Part model, mm, in its own coordinate system. Face numbers are marked on the shaded views. A direction names the side the tool comes from. Give positions to 0.01 mm unless a question says otherwise; leave off trailing zeros. Order: outer loops, then holes, each group sorted by start corner. A loop starts at its lowest first (then second) coordinate and runs counter-clockwise, first axis right, second up. Notation, with made-up numbers: M 25,80.25 L 58,80.25 A10 ccw 58,89.25 Z; hole C 38.5,-28 d1. An arc over 180 degrees is marked long. Answer as a JSON object with one key per item and string values.
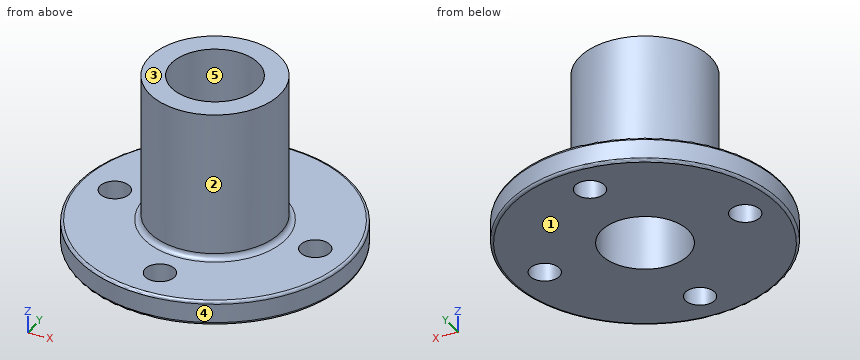
from build123d import *

# Parameters (mm, degrees)
CUT_EXTRUDE1_DEPTH      = 48.68647607
CUT_EXTRUDE1_DEPTH_BACK = 48.68647607
SKETCH2_R               = 2.7


with BuildPart() as part:
    # Sketch1 → Revolve1 (revolve)
    with BuildSketch(Plane(origin=(0, 0, 0), x_dir=(0, 0, -1), z_dir=(1, 0, 0)), mode=Mode.PRIVATE) as revolve1_sk:
        with BuildLine():
            Line((-16, 8), (16, 8))
            Line((16, 8), (16, 24.5))
            ThreePointArc((16, 24.5), (15.853553391, 24.853553391), (15.5, 25))
            Line((15.5, 25), (12, 25))
            ThreePointArc((12, 25), (11.646446609, 24.853553391), (11.5, 24.5))
            Line((11.5, 24.5), (11.5, 13))
            ThreePointArc((11.5, 13), (11.207106781, 12.292893219), (10.5, 12))
            Line((10.5, 12), (-16, 12))
            Line((-16, 12), (-16, 8))
        make_face()
    revolve(revolve1_sk.sketch.rotate(Axis((0, 0, 0), (0, 0, 1)), 90), axis=Axis((0, 0, 0), (0, 0, 1)))

    # Sketch2 → Cut-Extrude1 (cut, two sides: drawn at the far end of the back side and taken through both)
    with BuildSketch(Plane(origin=(0, 0, -16), x_dir=(-1, 0, 0), z_dir=(0, 0, -1)).offset(-CUT_EXTRUDE1_DEPTH_BACK)):
        with Locations((0, 18.5)):
            Circle(SKETCH2_R)
        with Locations((18.5, 0)):
            Circle(SKETCH2_R)
        with Locations((0, -18.5)):
            Circle(SKETCH2_R)
        with Locations((-18.5, 0)):
            Circle(SKETCH2_R)
    extrude(amount=CUT_EXTRUDE1_DEPTH + CUT_EXTRUDE1_DEPTH_BACK, mode=Mode.SUBTRACT)


solid = part.part
1. Probe line 1 along Y through (x, z) = (0, -12); line 2 along Y through (x, z) = (-2, 6); line 3 along Z through (x, y) = (11, -11). List the from-to ranges inside material, lowest first.
Worked answers:
{"line 1": "y = -25 to -21.2, -15.8 to -8, 8 to 15.8, 21.2 to 25", "line 2": "y = -11.83 to -7.75, 7.75 to 11.83", "line 3": "z = -16 to -11.5"}
2. Which spindle directions (+Z, -Z, +X, -X, +Y, -Y) get a long thin tool onto all of the face, cutting with end or side? Do the marked faces 1 and 2. Say none if no direction does.
Worked answers:
{"face 1": "-Z, +X, -X, +Y, -Y", "face 2": "+Z"}
3. Cut at A-A on x = 0. Give the cut face in (y, z), plus the area to 3 significant figures.
Worked answers:
{"outline": "M -25,-15.5 A0.5 ccw -24.5,-16 L -21.2,-16 L -21.2,-11.5 L -24.5,-11.5 A0.5 ccw -25,-12 Z; M -15.8,-16 L -8,-16 L -8,16 L -12,16 L -12,-10.5 A1 cw -13,-11.5 L -15.8,-11.5 Z; M 8,-16 L 15.8,-16 L 15.8,-11.5 L 13,-11.5 A1 cw 12,-10.5 L 12,16 L 8,16 Z; M 21.2,-16 L 24.5,-16 A0.5 ccw 25,-15.5 L 25,-12 A0.5 ccw 24.5,-11.5 L 21.2,-11.5 Z", "area": "325 mm^2"}
4. Two-plate mould, pull along Y, no slides. Class the marked faces 3, 4 and 5: +Y half, -Y half, draft (parallel to the pull), parting line (faces both ways), or undercut.
Worked answers:
{"face 3": "draft", "face 4": "parting line", "face 5": "undercut"}
5. Pin check, flat tips, straight feed: P1, Ø8.5, axis at x = -18.5, y = 0, coming from the +Z side; P2, Ø12, axis at x = -7.5, z = 4, coming from the -Y side; P3, Ø18.5, axis at x = 0, y = 0, coming from the +Z side; P4, Ø4, axis at y = -5, z = 1, coming from the -X side. Stop position of each tip, or through.
Worked answers:
{"P1": "stops at z = -11.5", "P2": "stops at y = -11.91", "P3": "stops at z = 16", "P4": "stops at x = -11.62"}
6. Cut at C-C on z = 4. Give the cut face in (x, y).
Worked answers:
{"outline": "C 0,0 d24; hole C 0,0 d16"}
